```python
from build123d import *

# Parameters (mm, degrees)
F1_DEPTH = 2
F3_DEPTH = 40
F5_DEPTH = 25


with BuildPart() as f1:
    # F0 (on Front) → F1 (new body)
    with BuildSketch(Plane.XZ):
        Polygon((35, -15), (35, 0), (-35, 0), (-35, -15), (-20, -30), (20, -30), align=None)
    extrude(amount=F1_DEPTH)

    # F2 (on face) → F3 (join)
    with BuildSketch(Plane(origin=(0, 0, 0), x_dir=(-1, 0, 0), z_dir=(0, 1, 0))):
        Polygon((33, -14.1715728753), (19.1715728753, -28), (-19.1715728753, -28), (-33, -14.1715728753), (-35, -14.1715728753), (-35, -15), (-20, -30), (20, -30), (35, -15), (35, 0), (33, 0), (33, -2), align=None)
    extrude(amount=F3_DEPTH)

    # F4 (on face) → F5 (join)
    with BuildSketch(Plane(origin=(0, 40, 0), x_dir=(-1, 0, 0), z_dir=(0, 1, 0))):
        Polygon((-19.1715728753, -28), (19.1715728753, -28), (33, -14.1715728753), (33, 0), (-35, 0), (-35, -14.1715728753), (-33, -14.1715728753), align=None)
        Polygon((33, -14.1715728753), (19.1715728753, -28), (-19.1715728753, -28), (-33, -14.1715728753), (-35, -14.1715728753), (-35, -15), (-20, -30), (20, -30), (35, -15), (35, 0), (33, 0), align=None)
    extrude(amount=F5_DEPTH)


solid = f1.part
```
Could you check a few things on this model? Use its own coordinates, in mm. A direction names the side the tool comes from. Coordinates: 2 decimals unless noted, no trailing zeros. Write each loop counter-clockwise with the first axis right and the second up, starting at its lowest first coordinate (ties: lowest second). Pieces come first, ordered by that corner, then holes. Notation, with made-up numbers: M -1,-7.75 L 9,-7.75 A14 cw 9,6.25 Z; hole C 55,41.5 d8. An arc over 180 degrees is marked long. Answer as CSV lines item,"result". Start each with the question number.
1) I want a section at D-D, the plane y = 5. Please give me the cut outline in (x, z).
2) I want a section at B-B, the plane x = -10.5. Please give me the cut outline in (y, z).
3) I want a section at C-C, the plane z = -26.75. Please give me the cut outline in (x, y), and give its area (3 significant figures).
4) I want a section at A-A, the plane z = -6.5. Please give me the cut outline in (x, y).
5) For faces 1 (the flat face through (-33, 20, -7)), 2 (the flat face through (-26.18, 19.72, -20.99)), 3 (the flat face through (0, -2, -15)), which set-ups out of +Z, -Z, +X, -X, +Y, -Y let a thin tool reach every point of the face, with its end or its side?
6) For P1, Ø8, axis at x = 21.5, y = 9.5, coming from the +Z side; P2, Ø2, axis at x = -26.5, y = 16, coming from the -Z side; P3, Ø4.5, axis at y = 25, z = -8.5, coming from the +X side, each with a flat end and sliding along its axis, tell me the tip position at first contact or that it passes through.
7) Please list where these lines run through material, in increasing order: line 1 (Y direction, x = -6.5, z = -22); line 2 (X direction, y = 5.5, z = -14.5); line 3 (X direction, y = 16, z = -16.25). Write a range as from..to.
8) We'd pull the mould along Y, two halves only. Please class faces 4 (the flat face through (28, 31, -22)), 5 (the flat face through (25.99, 19.72, -21.18)), 6 (the flat face through (1, 0, -14)), 7 (the flat face through (0, 65, -15)): +Y half, -Y half, draft (parallel to the pull), parting line (faces both ways), or undercut.
Data:
1,outline,"M -35,-15 L -20,-30 L 20,-30 L 35,-15 L 35,-14.17 L 33,-14.17 L 19.17,-28 L -19.17,-28 L -33,-14.17 L -33,0 L -35,0 Z"
2,outline,"M -2,-30 L 65,-30 L 65,0 L 40,0 L 40,-28 L 0,-28 L 0,0 L -2,0 Z"
3,outline,"M -23.25,-2 L 23.25,-2 L 23.25,65 L -23.25,65 Z; hole M -20.42,0 L 20.42,0 L 20.42,40 L -20.42,40 Z"
3,area,"1,480 mm^2"
4,outline,"M -35,-2 L 35,-2 L 35,0 L -33,0 L -33,40 L 35,40 L 35,65 L -35,65 Z"
5,face 1,"+Z, +X"
5,face 2,"+Z"
5,face 3,"+Z, -Z, +X, -X, -Y"
6,P1,"stops at z = -21.67"
6,P2,"stops at z = -24.5"
6,P3,"stops at x = -33"
7,line 1,"y = -2..0, 40..65"
7,line 2,"x = -35..-32.67, 32.67..35"
7,line 3,"x = -33.75..-30.92, 30.92..33.75"
8,face 4,"draft"
8,face 5,"undercut"
8,face 6,"undercut"
8,face 7,"+Y half"
